Geometry: see drawing. Coordinates: mm, zero at the bounding-box minimum. A direction names the side the tool comes from. Give positions to 0.01 mm unless a question says otherwise; leave off trailing zeros. Order: outer loops, then holes, each group sorted by start corner. A loop starts at its lowest first (then second) coordinate and runs counter-clockwise, first axis right, second up. Notation, with made-up numbers: (18, 25) - (52, 25) arc R17 cw to (52, 44) - close; hole circle Ø7 at (7.25, 33). An arc over 180 degrees is marked (long way). Write item = value, one per line. Start each with the question number.
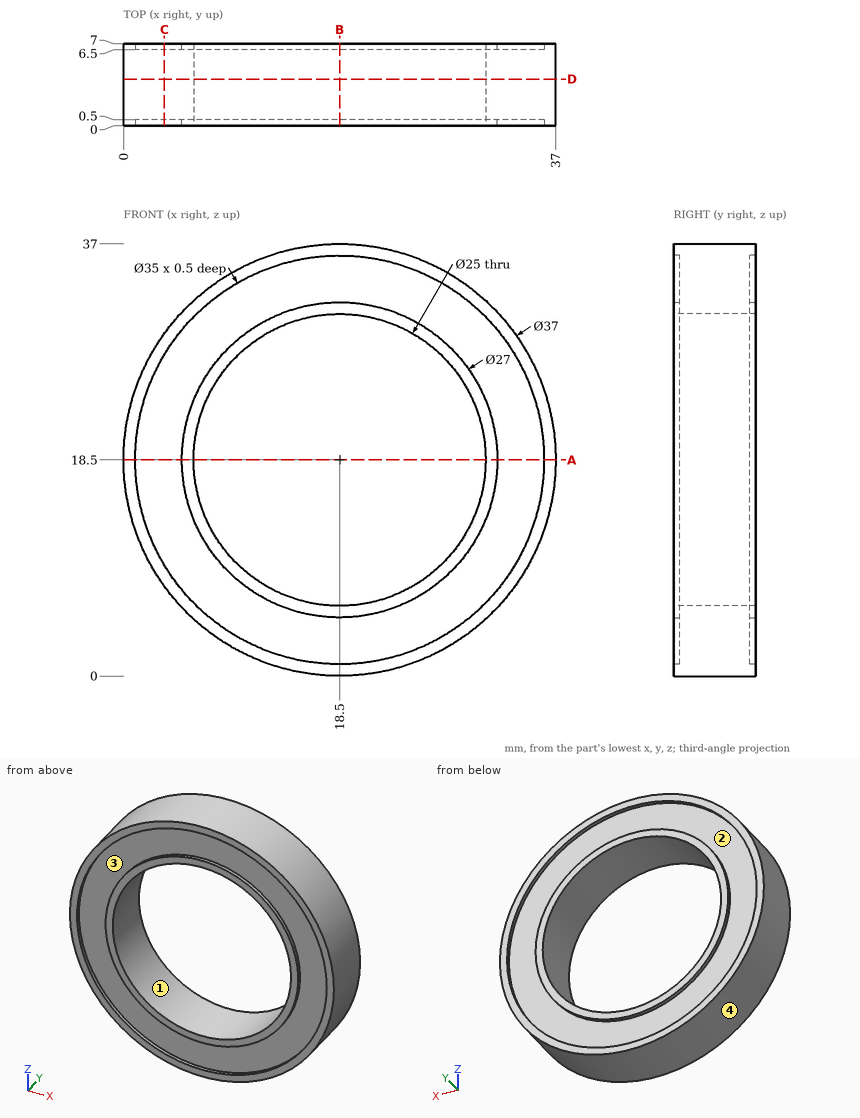
Q1. Section D-D, the plane y = 4. Return the cut outline in (x, z), then the cut area to 3 significant figures.
Q2. Pull-direction query (X, two-part tool) for the marked faces 3 and 4; classes: +X half, -X half, draft (parallel to the pull), parting line (faces both ways), or undercut.
Q3. Set-up query: the marked faces 1 and 2. Return all of +Z, -Z, +X, -X, +Y, -Y with unobstructed straight access to the full face (end or side cutting, diameter ignored); none if empty.
Q4. Contact query for flat-ended pins moving along their axis: pin 1 (2 mm diameter, centred on y = 3.5, z = 17, fed in from +X); pin 2 (1 mm diameter, centred on x = 26.5, y = 5.5, fed in from +Z); pin 3 (4 mm diameter, centred on y = 5, z = 8, fed in from +X); pin 4 (21 mm diameter, centred on x = 18.5, z = 18.5, fed in from +Y). Output: stop coordinate, or through.
Q5. Material intervals for line 1 along Z through (x, y) = (18.5, 0.3); line 2 along Y through (x, z) = (34, 19), sorted ascending. Write a range as from..to.
Q6. Section A-A, the plane z = 18.5. Return the cut outline in (x, y).
Q7. Section B-B, the plane x = 18.5. Return the cut outline in (y, z), then the cut area to 3 significant figures.
Q8. Section C-C, the plane x = 3.5. Return the cut outline in (y, z), then the cut area to 3 significant figures.
The answers:
q1.outline = circle Ø37 at (18.5, 18.5); hole circle Ø25 at (18.5, 18.5)
q1.area = 584 mm²
q2.face_3 = undercut
q2.face_4 = parting line
q3.face_1 = +Y, -Y
q3.face_2 = +Y
q4.pin_1 = 36.99
q4.pin_2 = 35.41
q4.pin_3 = 34.93
q4.pin_4 = through
q5.line_1 = 0..1, 5..6, 31..32, 36..37
q5.line_2 = 0.5..6.5
q6.outline = (0, 0) - (1, 0) - (1, 0.5) - (5, 0.5) - (5, 0) - (6, 0) - (6, 7) - (5, 7) - (5, 6.5) - (1, 6.5) - (1, 7) - (0, 7) - close; (31, 0) - (32, 0) - (32, 0.5) - (36, 0.5) - (36, 0) - (37, 0) - (37, 7) - (36, 7) - (36, 6.5) - (32, 6.5) - (32, 7) - (31, 7) - close
q7.outline = (0, 0) - (7, 0) - (7, 1) - (6.5, 1) - (6.5, 5) - (7, 5) - (7, 6) - (0, 6) - (0, 5) - (0.5, 5) - (0.5, 1) - (0, 1) - close; (0, 31) - (7, 31) - (7, 32) - (6.5, 32) - (6.5, 36) - (7, 36) - (7, 37) - (0, 37) - (0, 36) - (0.5, 36) - (0.5, 32) - (0, 32) - close
q7.area = 76.0 mm²
q8.outline = (0, 7.67) - (7, 7.67) - (7, 9.49) - (6.5, 9.49) - (6.5, 27.51) - (7, 27.51) - (7, 29.33) - (0, 29.33) - (0, 27.51) - (0.5, 27.51) - (0.5, 9.49) - (0, 9.49) - close
q8.area = 134 mm²
